Work out the finished part from the listing and answer in its coordinate system (mm). A direction names the side the tool comes from. Round coordinates to 2 decimals unless told otherwise and drop trailing zeros. Write each loop counter-clockwise with the first axis right and the second up, starting at its lowest first coordinate (ties: lowest second). Pieces come first, ordered by that corner, then holes. Notation, with made-up numbers: (-3.5, 55) - (26.5, 55) arc R20 ccw to (26.5, 88) - close; hole circle Ø8 at (-39, 27.5). An arc over 180 degrees is marked (long way). Write item = value, one per line. Start each with the question number.
from build123d import *

# Parameters (mm, degrees)
BOSS_EXTRUDE1_DEPTH = 14
SHELL1_T            = 2
SKETCH3_W           = 2
SKETCH3_H           = 50
SKETCH3_W_2         = 1.814522713
BOSS_EXTRUDE2_DEPTH = 2
SKETCH4_W           = 31.017616101
SKETCH4_H           = 3.530460369
BOSS_EXTRUDE3_DEPTH = 2


with BuildPart() as part:
    # Sketch1 → Boss-Extrude1 (new body)
    with BuildSketch(Plane(origin=(0, 0, 0), x_dir=(1, 0, 0), z_dir=(0, 1, 0))):
        Polygon((0, 0), (0, 56), (7.260584432, 56), (13.399361706, 60.750217247), (49.399361706, 60.750217247), (56, 56), (58, 56), (58, 0), align=None)
    extrude(amount=BOSS_EXTRUDE1_DEPTH)

    # Shell1
    shell1_openings = [part.faces().sort_by_distance(p)[0] for p in [
        (29.147078279, 14, -29.765448683),
    ]]
    offset(amount=SHELL1_T, openings=shell1_openings, kind=Kind.INTERSECTION)

    # Sketch3 → Boss-Extrude2 (add)
    with BuildSketch(Plane(origin=(0, 0, 0), x_dir=(1, 0, 0), z_dir=(0, 1, 0))):
        with Locations((1, 27.58353092)):
            Rectangle(SKETCH3_W, SKETCH3_H)
        with Locations((56.968981121, 27.58353092)):
            Rectangle(SKETCH3_W_2, SKETCH3_H)
    extrude(amount=BOSS_EXTRUDE2_DEPTH)

    # Sketch4 → Boss-Extrude3 (add)
    with BuildSketch(Plane(origin=(0, 0, 0), x_dir=(1, 0, 0), z_dir=(0, 1, 0))):
        with Locations((31.80262956, 58.741489624)):
            Rectangle(SKETCH4_W, SKETCH4_H)
    extrude(amount=BOSS_EXTRUDE3_DEPTH)


solid = part.part
1. For a pull along X with two mould halves and no side action, classify faces 3 (the face through (57, 1, -52.584)), 4 (the face through (29, -2, -31)), 5 (the face through (9.6, 5.89, -60.34)), 6 (the face through (53.298, 5.888, -60.408)) as released by +X, released by -X, zero draft, split by the parting line, or undercut.
2. Find section A-A on y = 9.5. Give the vertices of the cut face in (x, z).
3. Which of the six approach directions +Z, -Z, +X, -X, +Y, -Y give full straight-line access (tool end or side, diameter ignored) to faces 1 (the face through (32, 1, -60.507)), 2 (the face through (59, 14, -31))?
4. Find section D-D on x = 15. Give the vertices of the cut face in (y, z).
5. Consider line 1 (Z direction, x = 46.5, y = 0.5); line 2 (Z direction, x = 40, y = 8.5); line 3 (X direction, y = 10, z = -29). Determine where each line is inside the solid, lowest interval first.
6. Each of these flat-tipped pins is pushed along its axis until it touches: pin 1 (0.9 mm diameter, centred on x = 57, z = -34.5, fed in from +Y); pin 2 (3 mm diameter, centred on x = 38.5, z = -28.5, fed in from +Y); pin 3 (1 mm diameter, centred on x = 1.5, y = 1.5, fed in from -Z). Where does it stop, or does it pass through?
7. Find section B-B on x = 45. Give the vertices of the cut face in (y, z), plus the area to 3 significant figures.
8. Find section C-C on z = -30. Give the vertices of the cut face in (x, y), plus the area to 3 significant figures.
Answer key:
q1.face_3 = undercut
q1.face_4 = zero draft
q1.face_5 = released by -X
q1.face_6 = released by +X
q2.outline = (-2, -58) - (6.58, -58) - (12.72, -62.75) - (50.04, -62.75) - (56.64, -58) - (60, -58) - (60, 2) - (-2, 2) - close; hole (0, -56) - (7.26, -56) - (13.4, -60.75) - (49.4, -60.75) - (56, -56) - (58, -56) - (58, 0) - (0, 0) - close
q3.face_1 = +Y
q3.face_2 = +Z, -Z, +X, -X, +Y
q4.outline = (-2, -62.75) - (14, -62.75) - (14, -60.75) - (0, -60.75) - (0, 0) - (14, 0) - (14, 2) - (-2, 2) - close
q5.line_1 = -62.75 to -60.75, -60.51 to -56.98, 0 to 2
q5.line_2 = -62.75 to -60.75, 0 to 2
q5.line_3 = -2 to 0, 58 to 60
q6.pin_1 = 2
q6.pin_2 = 0
q6.pin_3 = -58
q7.outline = (-2, -62.75) - (14, -62.75) - (14, -60.75) - (0, -60.75) - (0, -60.51) - (2, -60.51) - (2, -56.98) - (0, -56.98) - (0, 0) - (14, 0) - (14, 2) - (-2, 2) - close
q7.area = 193 mm²
q8.outline = (-2, -2) - (60, -2) - (60, 14) - (58, 14) - (58, 0) - (57.88, 0) - (57.88, 2) - (56.06, 2) - (56.06, 0) - (2, 0) - (2, 2) - (0, 2) - (0, 14) - (-2, 14) - close
q8.area = 188 mm²
